```python
from build123d import *

# Parameters (mm, degrees)
SKETCH_1_R          = 4
EXTRUDE_1_DEPTH     = 40
CUT_EXTRUDE_START   = 5
SKETCH_2_R          = 10
CUT_EXTRUDE_1_DEPTH = 40


with BuildPart() as part:
    # 草图1 → 凸台-拉伸1 (new body)
    with BuildSketch(Plane.XY):
        with BuildLine():
            Line((8, 15), (30, 15))
            Line((30, 15), (30, -15))
            Line((30, -15), (-30, -15))
            Line((-30, -15), (-30, 5))
            Line((-30, 5), (5, 5))
            Line((5, 5), (5, 12))
            ThreePointArc((5, 12), (5.878679656, 14.121320344), (8, 15))
        make_face()
        with Locations((10, 0)):
            Circle(SKETCH_1_R, mode=Mode.SUBTRACT)
    extrude(amount=EXTRUDE_1_DEPTH)

    # 草图2 → 切除-拉伸1 (cut)
    with BuildSketch(Plane(origin=(0, 0, 0), x_dir=(1, 0, 0), z_dir=(0, 1, 0)).offset(CUT_EXTRUDE_START)):
        with Locations(Location((-12.5, -20, 0), (0, 0, 270))):
            Circle(SKETCH_2_R)
    extrude(amount=-CUT_EXTRUDE_1_DEPTH, mode=Mode.SUBTRACT)


solid = part.part
```
Check sheet for the modelled part. Datum: model origin and axes. Units: mm. A direction names the side the tool comes from. Round coordinates to 2 decimals unless told otherwise and drop trailing zeros. Loops run counter-clockwise (first coordinate to the right, second up) from the corner with the lowest first, then second, coordinate; pieces in that order, holes last. Notation, with made-up numbers: (51, 24) - (79, 24) arc R35 ccw to (79, 61) - close; hole circle Ø2 at (-2, 33.5). An arc over 180 degrees is marked (long way). Write item = value, one per line. Start each with the question number.
Q1. Section check B-B (z = 20). Record the boundary of the cut face in (x, y).
Q2. Section check A-A (y = 0). Record the boundary of the cut face in (x, z), plus the area to 3 significant figures.
Q3. Section check C-C (x = 10). Record the boundary of the cut face in (y, z).
Q4. Access from +Z, -Z, +X, -X, +Y, -Y to the whole of each face (thin tool, end or side, straight path). Record for faces 1 (the face through (19, 15, 20)), 2 (the face through (5, 8, 20)).
Q5. Thickness scan on L1, parallel to Y at x = 10, z = 20; L2, parallel to X at y = -6.25, z = 20.5; L3, parallel to Y at x = -15.5, z = 35. Record the ranges inside material, lowest first.
Q6. Section check D-D (y = -5.5). Record the boundary of the cut face in (x, z), plus the area to 3 significant figures.
Q7. Release check for a two-part mould opening along Z. For faces 3 (the face through (-9.5, -4.86, 29.54)), 4 (the face through (30, 0, 20)), 5 (the face through (0, -3, 0)), 6 (the face through (0, -3, 40)) record: pulls with the +Z half, pulls with the -Z half, needs draft (parallel to the pull), parting line crosses it, or undercut.
Q8. Depth check by flat-ended pin: P1, Ø10.5, axis at x = 10, y = 0, coming from the -Z side; P2, Ø5, axis at y = 9, z = 30.5, coming from the -X side; P3, Ø23, axis at x = -12.5, z = 20, coming from the +Y side. Enter the tip coordinate at first touch or a pass-through.
Derived:
q1.outline = (-30, -15) - (-22.5, -15) - (-22.5, 5) - (-30, 5) - close; (-2.5, -15) - (30, -15) - (30, 15) - (8, 15) arc R3 ccw to (5, 12) - (5, 5) - (-2.5, 5) - close; hole circle Ø8 at (10, 0)
q2.outline = (-30, 0) - (6, 0) - (6, 40) - (-30, 40) - close; (14, 0) - (30, 0) - (30, 40) - (14, 40) - close; hole circle Ø20 at (-12.5, 20)
q2.area = 1,770 mm^2
q3.outline = (-15, 0) - (-4, 0) - (-4, 40) - (-15, 40) - close; (4, 0) - (15, 0) - (15, 40) - (4, 40) - close
q4.face_1 = +Z, -Z, +X, -X, +Y
q4.face_2 = +Z, -Z, -X, +Y
q5.L1 = -15 to -4, 4 to 15
q5.L2 = -30 to -22.49, -2.51 to 30
q5.L3 = -15 to 5
q6.outline = (-30, 0) - (30, 0) - (30, 40) - (-30, 40) - close; hole circle Ø20 at (-12.5, 20)
q6.area = 2,090 mm^2
q7.face_3 = undercut
q7.face_4 = needs draft
q7.face_5 = pulls with the -Z half
q7.face_6 = pulls with the +Z half
q8.P1 = 0
q8.P2 = 5
q8.P3 = 5
